from build123d import *

# Parameters (mm, degrees)
SKETCH1_R           = 1.5
BOSS_EXTRUDE1_DEPTH = 1
BOSS_EXTRUDE2_DEPTH = 3.5
BOSS_EXTRUDE3_DEPTH = 0.5
SKETCH4_R           = 0.25
CUT_EXTRUDE1_DEPTH  = 38.70941527


with BuildPart() as part:
    # Sketch1 → Boss-Extrude1 (new, symmetric)
    with BuildSketch(Plane(origin=(0, 0, 0), x_dir=(1, 0, 0), z_dir=(0, 1, 0))):
        with BuildLine():
            Line((-15, -18), (15, -18))
            ThreePointArc((15, -18), (17.121320344, -17.121320344), (18, -15))
            Line((18, -15), (18, 15))
            ThreePointArc((18, 15), (17.121320344, 17.121320344), (15, 18))
            Line((15, 18), (-15, 18))
            ThreePointArc((-15, 18), (-17.121320344, 17.121320344), (-18, 15))
            Line((-18, 15), (-18, -15))
            ThreePointArc((-18, -15), (-17.121320344, -17.121320344), (-15, -18))
        make_face()
        with Locations(Location((15.25, 15.25, 0), (0, 0, 270))):
            Circle(SKETCH1_R, mode=Mode.SUBTRACT)
        with Locations(Location((-15.25, 15.25, 0), (0, 0, 90))):
            Circle(SKETCH1_R, mode=Mode.SUBTRACT)
        with Locations(Location((15.25, -15.25, 0), (0, 0, 90))):
            Circle(SKETCH1_R, mode=Mode.SUBTRACT)
        with Locations(Location((-15.25, -15.25, 0), (0, 0, 270))):
            Circle(SKETCH1_R, mode=Mode.SUBTRACT)
    extrude(amount=BOSS_EXTRUDE1_DEPTH, both=True)

    # Sketch2 → Boss-Extrude2 (add)
    with BuildSketch(Plane.XY.offset(18)):
        with BuildLine():
            Line((-8, 1), (-4, 1))
            Line((-4, 1), (-4, 2.408392022))
            ThreePointArc((-4, 2.408392022), (-4.023623738, 2.472941744), (-4.083333333, 2.506993351))
            ThreePointArc((-4.083333333, 2.506993351), (-4.353553391, 2.646446609), (-4.493006649, 2.916666667))
            ThreePointArc((-4.493006649, 2.916666667), (-4.527058256, 2.976376262), (-4.591607978, 3))
            Line((-4.591607978, 3), (-7.408392022, 3))
            ThreePointArc((-7.408392022, 3), (-7.472941744, 2.976376262), (-7.506993351, 2.916666667))
            ThreePointArc((-7.506993351, 2.916666667), (-7.646446609, 2.646446609), (-7.916666667, 2.506993351))
            ThreePointArc((-7.916666667, 2.506993351), (-7.976376262, 2.472941744), (-8, 2.408392022))
            Line((-8, 2.408392022), (-8, 1))
        make_face()
        with BuildLine():
            Line((-4.1, 1.1), (-4.1, 2.408392022))
            ThreePointArc((-4.1, 2.408392022), (-4.424264069, 2.575735931), (-4.591607978, 2.9))
            Line((-4.591607978, 2.9), (-7.408392022, 2.9))
            ThreePointArc((-7.408392022, 2.9), (-7.575735931, 2.575735931), (-7.9, 2.408392022))
            Line((-7.9, 2.408392022), (-7.9, 1.1))
            Line((-7.9, 1.1), (-4.1, 1.1))
        make_face(mode=Mode.SUBTRACT)
    extrude(amount=-BOSS_EXTRUDE2_DEPTH)

    # Sketch3 → Boss-Extrude3 (add)
    with BuildSketch(Plane(origin=(0, 0, 14.5), x_dir=(-1, 0, 0), z_dir=(0, 0, -1))):
        with BuildLine():
            Line((8, 1), (8, 2.408392022))
            ThreePointArc((8, 2.408392022), (7.976376262, 2.472941744), (7.916666667, 2.506993351))
            ThreePointArc((7.916666667, 2.506993351), (7.646446609, 2.646446609), (7.506993351, 2.916666667))
            ThreePointArc((7.506993351, 2.916666667), (7.472941744, 2.976376262), (7.408392022, 3))
            Line((7.408392022, 3), (4.591607978, 3))
            ThreePointArc((4.591607978, 3), (4.527058256, 2.976376262), (4.493006649, 2.916666667))
            ThreePointArc((4.493006649, 2.916666667), (4.353553391, 2.646446609), (4.083333333, 2.506993351))
            ThreePointArc((4.083333333, 2.506993351), (4.023623738, 2.472941744), (4, 2.408392022))
            Line((4, 2.408392022), (4, 1))
            Line((4, 1), (8, 1))
        make_face()
    extrude(amount=-BOSS_EXTRUDE3_DEPTH)

    # Sketch4 → Cut-Extrude1 (cut, through all)
    with BuildSketch(Plane.XY.offset(15)):
        with Locations((-7, 2.6)):
            Circle(SKETCH4_R)
        with Locations((-6, 2.6)):
            Circle(SKETCH4_R)
        with Locations((-5, 2.6)):
            Circle(SKETCH4_R)
    extrude(amount=-CUT_EXTRUDE1_DEPTH, mode=Mode.SUBTRACT)


solid = part.part
The listing builds one solid part. Answer for the finished solid, in the listing's coordinates (mm). A direction names the side the tool comes from. Give positions to 0.01 mm unless a question says otherwise; leave off trailing zeros. Write each loop counter-clockwise with the first axis right and the second up, starting at its lowest first coordinate (ties: lowest second). Pieces come first, ordered by that corner, then holes.
1) Section A-A (z = -16) is taken. Write down the section's boundary in (x, y), and give its area (3 significant figures).
2) For a pull along X with two mould halves and no side action, classify faces 3 (the face through (-6, 2, 14.5)), 4 (the face through (-17.14, 0.01, 17.1)), 5 (the face through (15.18, -0.01, 16.75)) as pulls with the +X half, pulls with the -X half, needs draft (parallel to the pull), parting line crosses it, or undercut.
3) Section C-C (z = -11) is taken. Write down the section's boundary in (x, y), and give its area (3 significant figures).
4) A tool of negligible diameter and unlimited length cuts with its end or side. For faces 1 (the face through (-17.1, 0.01, -17.14)), 2 (the face through (-6, 2, 15)), from which of +Z, -Z, +X, -X, +Y, -Y can it reach the whole face along a straight path? Write none if from no direction.
5) Given P1, Ø0.7, axis at y = 2, z = 16.5, coming from the +X side; P2, Ø1, axis at y = 2, z = -13.5, coming from the -X side; P3, Ø2, axis at x = -5.5, y = 2.5, coming from the -Z side; P4, Ø11, axis at x = -7, z = -7, coming from the +Y side, each flat-ended and moving along its own axis, determine where each tip first touches the part or whether it passes through.
6) Find the intervals of material crossed by L1, parallel to X at y = 0.4, z = 15.25; L2, parallel to Y at x = -5, z = 14.7; L3, parallel to Y at x = -8, z = -12, in increasing order.
7) Section B-B (x = -2) is taken. Write down the section's boundary in (y, z).
Response:
1. outline: (-17.83, -1) - (-16.55, -1) - (-16.55, 1) - (-17.83, 1) - close; (-13.95, -1) - (13.95, -1) - (13.95, 1) - (-13.95, 1) - close; (16.55, -1) - (17.83, -1) - (17.83, 1) - (16.55, 1) - close
1. area: 60.9 mm2
2. face 3: needs draft
2. face 4: pulls with the -X half
2. face 5: undercut
3. outline: (-18, -1) - (18, -1) - (18, 1) - (-18, 1) - close
3. area: 72.0 mm2
4. face 1: -Z, -X, +Y, -Y
4. face 2: +Z
5. P1: stops at x = -4
5. P2: passes through
5. P3: stops at z = 14.5
5. P4: stops at y = 1
6. L1: x = -17.99 to -16.75, -13.75 to 13.75, 16.75 to 17.99
6. L2: y = -1 to 2.35, 2.85 to 3
6. L3: y = -1 to 1
7. outline: (-1, -18) - (1, -18) - (1, 18) - (-1, 18) - close
